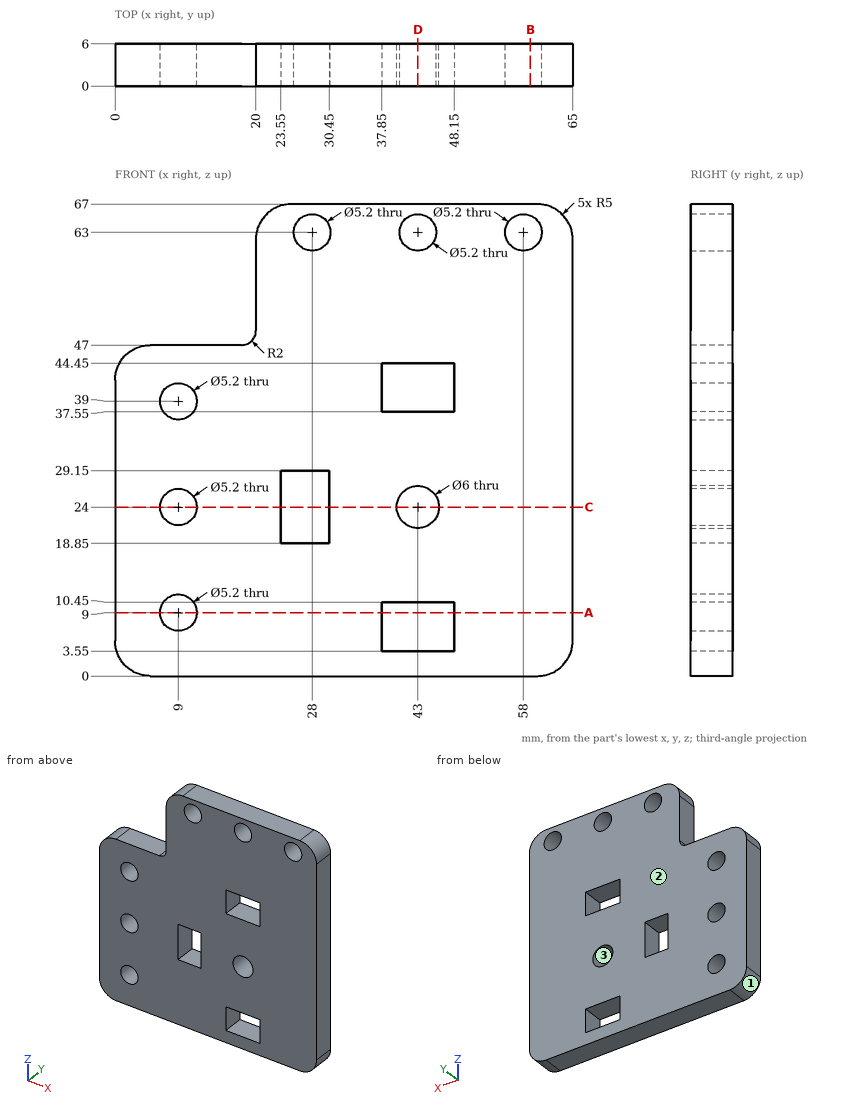
Here's the drawing with two shaded views (mm, measured from the low corner). I have some questions. Round coordinates to 2 decimals unless told otherwise and drop trailing zeros. Loops run counter-clockwise (first coordinate to the right, second up) from the corner with the lowest first, then second, coordinate; pieces in that order, holes last.
1. Will this pin go through, and if not, where does the flat tip stop? pin 1 (6 mm diameter, centred on x = 9, z = 39, fed in from +Y).
Answers:
pin 1: stops at y = 6
2. Thinking about a two-plate mould opening in X: for the marked faces 1, 2 and 3, which applies, released by +X, released by -X, zero draft, split by the parting line, or undercut?
Answers:
face 1: released by -X
face 2: zero draft
face 3: undercut
3. If I drill on probe 1 along X at (y, z) = (4.1, 9); probe 2 along Z at (x, y) = (47, 4.55); probe 3 along X at (y, z) = (4.4, 63), over which ranges is the centre line in solid material (lowest first)?
Answers:
probe 1: x = 0 to 6.4, 11.6 to 37.85, 48.15 to 65
probe 2: z = 0 to 3.55, 10.45 to 37.55, 44.45 to 67
probe 3: x = 20.1 to 25.4, 30.6 to 40.4, 45.6 to 55.4, 60.6 to 64.9
4. Suppose I cut it at D-D, the plane x = 43. Please give me the cut outline in (y, z).
Answers:
outline: (0, 0) - (6, 0) - (6, 3.55) - (0, 3.55) - close; (0, 10.45) - (6, 10.45) - (6, 21) - (0, 21) - close; (0, 27) - (6, 27) - (6, 37.55) - (0, 37.55) - close; (0, 44.45) - (6, 44.45) - (6, 60.4) - (0, 60.4) - close; (0, 65.6) - (6, 65.6) - (6, 67) - (0, 67) - close
5. Suppose I cut it at B-B, the plane x = 59. Please give me the cut outline in (y, z), and give its area (3 significant figures).
Answers:
outline: (0, 0) - (6, 0) - (6, 60.6) - (0, 60.6) - close; (0, 65.4) - (6, 65.4) - (6, 67) - (0, 67) - close
area: 373 mm2
6. Suppose I cut it at A-A, the plane z = 9. Please give me the cut outline in (x, y), and give its area (3 significant figures).
Answers:
outline: (0, 0) - (6.4, 0) - (6.4, 6) - (0, 6) - close; (11.6, 0) - (37.85, 0) - (37.85, 6) - (11.6, 6) - close; (48.15, 0) - (65, 0) - (65, 6) - (48.15, 6) - close
area: 297 mm2
7. Suppose I cut it at C-C, the plane z = 24. Please give me the cut outline in (x, y).
Answers:
outline: (0, 0) - (6.4, 0) - (6.4, 6) - (0, 6) - close; (11.6, 0) - (23.55, 0) - (23.55, 6) - (11.6, 6) - close; (30.45, 0) - (40, 0) - (40, 6) - (30.45, 6) - close; (46, 0) - (65, 0) - (65, 6) - (46, 6) - close
